Check sheet for the modelled part. Datum: model origin and axes. Units: mm. A direction names the side the tool comes from. Give positions to 0.01 mm unless a question says otherwise; leave off trailing zeros. Loops run counter-clockwise (first coordinate to the right, second up) from the corner with the lowest first, then second, coordinate; pieces in that order, holes last. Notation, with made-up numbers: M 51.25,81 L 107.25,81 A30 cw 107.25,104 Z; hole C 46.5,9.5 d1. An arc over 180 degrees is marked long. Use one line per item in the form item = value.
from build123d import *

# Parameters (mm, degrees)
F0_W     = 43.7379740179
F0_H     = 75.0739984214
F1_DEPTH = 2.54
F2_W     = 35.6321558356
F2_H     = 75.0739984214
F3_DEPTH = 6.604
F4_W     = 44.1027786583
F4_H     = 75.3439329565
F5_DEPTH = 4.572


# Not quite as in the source:
# - the program builds the solid bodies; features that only make, move or delete a surface that nothing else refers to are left out


with BuildPart() as f1:
    # F0 (on Right) → F1 (new body)
    with BuildSketch(Plane.YZ):
        with Locations((-2.128392458, 14.8043204099)):
            Rectangle(F0_W, F0_H)
    extrude(amount=F1_DEPTH)

    # F2 (on face) → F3 (join)
    with BuildSketch(Plane.YZ.offset(2.54)):
        with Locations((-6.1813015491, 14.8043204099)):
            Rectangle(F2_W, F2_H)
    extrude(amount=F3_DEPTH)

    # F4 (on face) → F5 (join)
    with BuildSketch(Plane.YZ.offset(9.144)):
        with Locations((-1.9459901378, 14.8043166846)):
            Rectangle(F4_W, F4_H)
    extrude(amount=F5_DEPTH)


solid = f1.part
1) Scan lines: line 1 (Z direction, x = 7, y = -15.5); line 2 (Y direction, x = 8.25, z = 31.5); line 3 (Y direction, x = 1.5, z = -5.5). Record each from-to range of solid material in increasing order.
Evaluation:
line_1 = -22.73 to 52.34
line_2 = -24 to 11.63
line_3 = -24 to 19.74
2) Section check A-A (z = 18). Record the cut outline in (x, y).
Evaluation:
outline = M 0,-24 L 13.72,-24 L 13.72,20.11 L 9.14,20.11 L 9.14,11.63 L 2.54,11.63 L 2.54,19.74 L 0,19.74 Z
3) Depth check by flat-ended pin: pin 1 Ø3 at (y, z) = (11.5, -12) entering from -X; pin 2 Ø5.5 at (x, z) = (5.5, 13) entering from +Y; pin 3 Ø4.5 at (x, y) = (6.5, 5.5) entering from +Z; pin 4 Ø7.5 at (x, y) = (4, -9) entering from -Z. Enter the tip coordinate at first touch or a pass-through.
Evaluation:
pin_1 = 0
pin_2 = 11.63
pin_3 = 52.34
pin_4 = -22.73
4) Set-up check for faces 4 (the face through (11, 20.105, 14)), 5 (the face through (1, 19.741, 14)), 6 (the face through (5, -7, 52.341)), 7 (the face through (6, 11.635, 14)), 8 (the face through (5, -7, -22.733)): record each of +Z, -Z, +X, -X, +Y, -Y from which the full face is reachable in a straight line by a thin tool's end or side.
Evaluation:
face_4 = +Z, -Z, +X, -X, +Y
face_5 = +Z, -Z, -X, +Y
face_6 = +Z, -X, +Y, -Y
face_7 = +Z, -Z, +Y
face_8 = -Z, -X, +Y, -Y
5) Release check for a two-part mould opening along X. For faces 1 (the face through (9.144, 16, 15)), 2 (the face through (13.716, -2, 15)), 3 (the face through (11, -2, 52.476)) record: pulls with the +X half, pulls with the -X half, needs draft (parallel to the pull), parting line crosses it, or undercut.
Evaluation:
face_1 = undercut
face_2 = pulls with the +X half
face_3 = needs draft
6) Section check B-B (x = 5.5). Record the cut outline in (y, z).
Evaluation:
outline = M -24,-22.73 L 11.63,-22.73 L 11.63,52.34 L -24,52.34 Z
